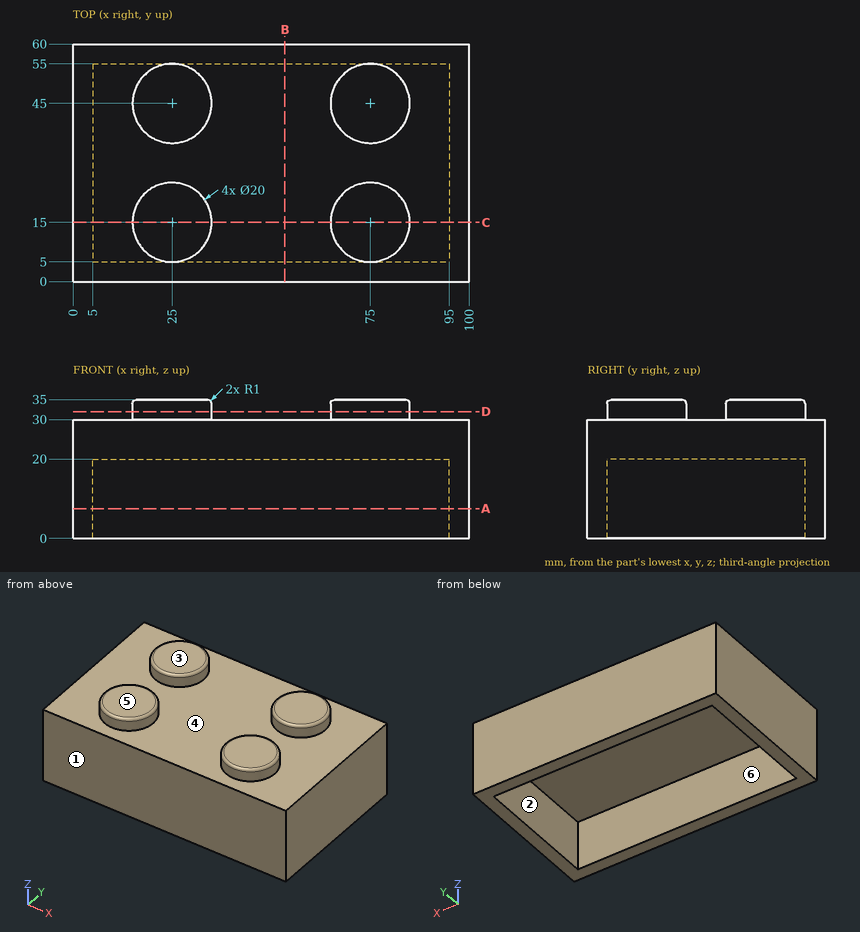
The drawing under review shows one solid part. Ordinate dimensions are in mm from its lowest x, y, z. A direction names the side the tool comes from. Round coordinates to 2 decimals unless told otherwise and drop trailing zeros. Write each loop counter-clockwise with the first axis right and the second up, starting at its lowest first coordinate (ties: lowest second). Pieces come first, ordered by that corner, then holes. Notation, with made-up numbers: (17.5, 12) - (41.5, 12) arc R18 ccw to (41.5, 34) - close; hole circle Ø5 at (51.25, 84). An arc over 180 degrees is marked (long way). Use one line per item in the form item = value.
Q1. Consider section A-A (z = 7.5). State the section outline as (x, y) points, and give its area (3 significant figures).
Answer key:
outline = (0, 0) - (100, 0) - (100, 60) - (0, 60) - close; hole (5, 5) - (95, 5) - (95, 55) - (5, 55) - close
area = 1,500 mm2
Q2. Consider section B-B (x = 53.5). State the section outline as (y, z) points, and give its area (3 significant figures).
Answer key:
outline = (0, 0) - (5, 0) - (5, 20) - (55, 20) - (55, 0) - (60, 0) - (60, 30) - (0, 30) - close
area = 800 mm2
Q3. Consider section D-D (z = 32). State the section outline as (x, y) points, and give its area (3 significant figures).
Answer key:
outline = circle Ø20 at (25, 15); circle Ø20 at (25, 45); circle Ø20 at (75, 15); circle Ø20 at (75, 45)
area = 1,260 mm2
Q4. Draft analysis for pull direction Y (two halves, no side actions). For the marked faces 1, 2 and 3, state which applies: +Y half, -Y half, draft (parallel to the pull), parting line (faces both ways), or undercut.
Answer key:
face_1 = -Y half
face_2 = undercut
face_3 = draft
Q5. Consider section C-C (y = 15). State the section outline as (x, z) points, and give its area (3 significant figures).
Answer key:
outline = (0, 0) - (5, 0) - (5, 20) - (95, 20) - (95, 0) - (100, 0) - (100, 30) - (85, 30) - (85, 34) arc R1 ccw to (84, 35) - (66, 35) arc R1 ccw to (65, 34) - (65, 30) - (35, 30) - (35, 34) arc R1 ccw to (34, 35) - (16, 35) arc R1 ccw to (15, 34) - (15, 30) - (0, 30) - close
area = 1,400 mm2
Q6. Insertion check: pin 1 Ø15 at (x, y) = (48.5, 38) entering from -Z; pin 2 Ø6 at (x, y) = (38.5, 13.5) entering from +Z. Each pin has a flat end and moves straight along its axis. Give the tip position at first contact, or say it passes through.
Answer key:
pin_1 = 20
pin_2 = 30
Q7. For line 1 (Y direction, x = 52.5, z = 19.5); line 2 (X direction, y = 28, z = 11.5); line 3 (Z direction, x = 56, y = 27), list the stretches that pass through material, from the lowest coordinate up. Write a range as [from, to].
Answer key:
line_1 = [0, 5], [55, 60]
line_2 = [0, 5], [95, 100]
line_3 = [20, 30]
Q8. Tool access review of the marked faces 4, 5 and 6: name each direction out of +Z, -Z, +X, -X, +Y, -Y from which nothing blocks a thin tool from reaching the whole face with its end or side.
Answer key:
face_4 = +Z
face_5 = +Z, +X, -X, +Y, -Y
face_6 = -Z
